Input: dimensioned drawing with shaded views. Units: mm. Origin: part minimum x, y, z. A direction names the side the tool comes from. Coordinates: 2 decimals unless noted, no trailing zeros. Order: outer loops, then holes, each group sorted by start corner. A loop starts at its lowest first (then second) coordinate and runs counter-clockwise, first axis right, second up. Notation, with made-up numbers: (-18, -6.5) - (6, -6.5) arc R17 ccw to (6, 16.5) - close; hole circle Ø8 at (71.5, 21). An arc over 180 degrees is marked (long way). Answer as CSV lines item,"result". Start each with the question number.
Item 1: Section A-A (z = 5). Output: boundary loops of the cut face in (x, y).
Item 2: Section B-B (y = 34). Output: boundary loops of the cut face in (x, z), and give its area (3 significant figures).
Item 3: Access query for the marked faces 4 and 5. Directions: +Z, -Z, +X, -X, +Y, -Y. A direction counts if a zero-diameter tool reaches every point of the face in a straight line with its end or side. Return the directions, or none.
Item 4: Section D-D (x = 16.5). Output: boundary loops of the cut face in (y, z).
Item 5: Material intervals for line 1 along Y through (x, z) = (9.5, 1.35); line 2 along Y through (x, z) = (14.75, 5.5); line 3 along X through (y, z) = (7.5, 0.95), sorted ascending.
Item 6: First-contact query: pin 1 (1 mm diameter, centred on x = 8.5, y = 12.5, fed in from +Z). Flat tip, straight axial feed; report the tip coordinate or a pass-through.
Item 7: Draft query along Y for the marked faces 1, 2 and 3. Return one class per face: +Y half, -Y half, draft (parallel to the pull), parting line (faces both ways), or undercut.
Item 8: Section C-C (x = 9.5). Output: boundary loops of the cut face in (y, z), and give its area (3 significant figures).
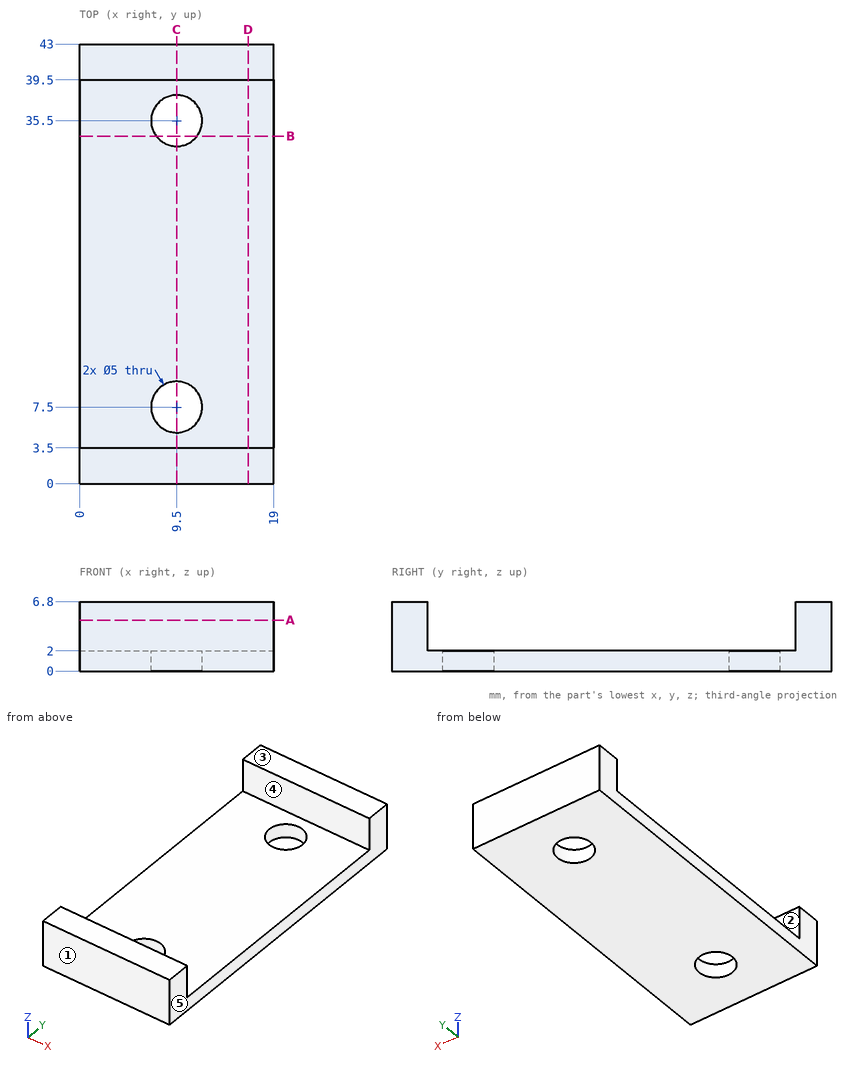
Determined:
1,outline,"(0, 0) - (19, 0) - (19, 3.5) - (0, 3.5) - close; (0, 39.5) - (19, 39.5) - (19, 43) - (0, 43) - close"
2,outline,"(0, 0) - (7.5, 0) - (7.5, 2) - (0, 2) - close; (11.5, 0) - (19, 0) - (19, 2) - (11.5, 2) - close"
2,area,"30.0 mm^2"
3,face 4,"+Z, +X, -X"
3,face 5,"+Z, -Z, +X, +Y, -Y"
4,outline,"(0, 0) - (43, 0) - (43, 6.8) - (39.5, 6.8) - (39.5, 2) - (3.5, 2) - (3.5, 6.8) - (0, 6.8) - close"
5,line 1,"y = 0 to 5, 10 to 33, 38 to 43"
5,line 2,"y = 0 to 3.5, 39.5 to 43"
5,line 3,"x = 0 to 7, 12 to 19"
6,pin 1,"stops at z = 2"
7,face 1,"-Y half"
7,face 2,"undercut"
7,face 3,"draft"
8,outline,"(0, 0) - (5, 0) - (5, 2) - (3.5, 2) - (3.5, 6.8) - (0, 6.8) - close; (10, 0) - (33, 0) - (33, 2) - (10, 2) - close; (38, 0) - (43, 0) - (43, 6.8) - (39.5, 6.8) - (39.5, 2) - (38, 2) - close"
8,area,"99.6 mm^2"
